For this review, take the finished solid that the model builds, in its own axes (mm). Face numbers are marked on the shaded views. A direction names the side the tool comes from. Coordinates: 2 decimals unless noted, no trailing zeros. Loops run counter-clockwise (first coordinate to the right, second up) from the corner with the lowest first, then second, coordinate; pieces in that order, holes last. Notation, with made-up numbers: M 41.25,29.5 L 62.25,29.5 A8 ccw 62.25,39.5 Z; hole C 77.25,-16 d4. An arc over 180 degrees is marked long. Use one line per item in the form item = value.
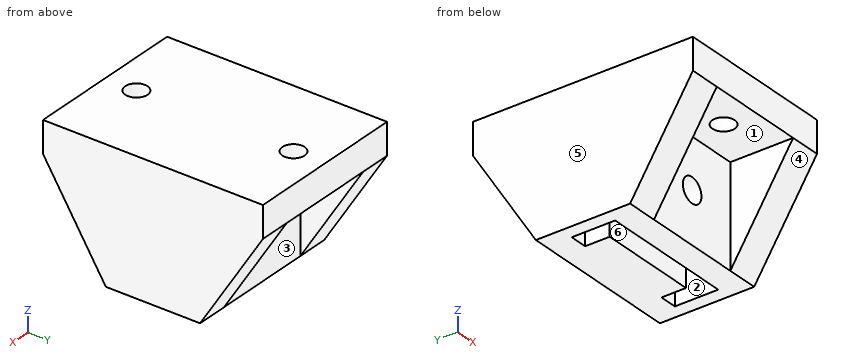
```python
from build123d import *

# Parameters (mm, degrees)
ESQUISSE1_W             = 33.02
ESQUISSE1_H             = 19.05
BOSS_EXTRU_1_DEPTH      = 20.32
ESQUISSE2_R             = 2.4765
ENL_V_MAT_EXTRU_1_DEPTH = 33.378773911
ESQUISSE3_W             = 33.02
ESQUISSE3_H             = 44.45
BOSS_EXTRU_2_DEPTH      = 6.35
BOSS_EXTRU_3_DEPTH      = 6.35
ESQUISSE6_R             = 2.25
ENL_V_MAT_EXTRU_2_DEPTH = 35.342875899


with BuildPart() as part:
    # Esquisse1 → Boss.-Extru.1 (new body)
    with BuildSketch(Plane.XY):
        Rectangle(ESQUISSE1_W, ESQUISSE1_H)
        Polygon((-13.716, 4.3815), (-13.716, -4.3815), (13.716, -4.3815), (13.716, 4.3815), (10.16, 4.3815), (10.16, -0.5715), (-10.16, -0.5715), (-10.16, 4.3815), align=None, mode=Mode.SUBTRACT)
    extrude(amount=BOSS_EXTRU_1_DEPTH)

    # Esquisse2 → Enlèv. mat.-Extru.1 (cut, through all)
    with BuildSketch(Plane(origin=(0, 9.525, 0), x_dir=(1, 0, 0), z_dir=(0, 1, 0))):
        with Locations(Location((0, -10.287, 0), (0, 0, 270))):
            Circle(ESQUISSE2_R)
    extrude(amount=-ENL_V_MAT_EXTRU_1_DEPTH, mode=Mode.SUBTRACT)

    # Esquisse3 → Boss.-Extru.2 (add)
    with BuildSketch(Plane.XY.offset(20.32)):
        Rectangle(ESQUISSE3_W, ESQUISSE3_H)
    extrude(amount=BOSS_EXTRU_2_DEPTH)

    # Esquisse5 → Boss.-Extru.3 (add)
    with BuildSketch(Plane(origin=(16.51, 0, 0), x_dir=(0, 0, -1), z_dir=(1, 0, 0))):
        Polygon((-20.32, -22.225), (0, -9.525), (-20.32, -9.525), align=None)
        Polygon((-20.32, 22.225), (0, 9.525), (-20.32, 9.525), align=None)
    boss_extru_3 = extrude(amount=-BOSS_EXTRU_3_DEPTH)

    # Symétrie1: Boss.-Extru.3 across plane
    add(boss_extru_3.mirror(Plane(origin=(0, 0, 0), x_dir=(0, 0, 1), z_dir=(1, 0, 0))))

    # Esquisse6 → Enlèv. mat.-Extru.2 (cut, through all)
    with BuildSketch(Plane(origin=(0, 0, 20.32), x_dir=(-1, 0, 0), z_dir=(0, 0, -1))):
        with Locations((0, -15.875)):
            Circle(ESQUISSE6_R)
        with Locations(Location((0, 15.875, 0), (0, 0, 180))):
            Circle(ESQUISSE6_R)
    extrude(amount=-ENL_V_MAT_EXTRU_2_DEPTH, mode=Mode.SUBTRACT)


solid = part.part
```
1. Consider section B-B on y = 2. Write out the cut boundary in (x, z).
Computed values:
outline = M -16.51,0 L -13.72,0 L -13.72,20.32 L -10.16,20.32 L -10.16,0 L 10.16,0 L 10.16,20.32 L 13.72,20.32 L 13.72,0 L 16.51,0 L 16.51,26.67 L -16.51,26.67 Z; hole C 0,10.29 d4.95
2. Consider section D-D on x = -13. Write out the cut boundary in (y, z) (1 decimal), plus the area to 3 significant figures.
Computed values:
outline = M -22.2,20.3 L -9.5,0 L -4.4,0 L -4.4,20.3 L 4.4,20.3 L 4.4,0 L 9.5,0 L 22.2,20.3 L 22.2,26.7 L -22.2,26.7 Z
area = 749 mm2
3. Consider section A-A on x = 0. Write out the cut boundary in (y, z) (1 decimal), plus the area to 3 significant figures.
Computed values:
outline = M -22.2,20.3 L -18.1,20.3 L -18.1,26.7 L -22.2,26.7 Z; M -13.6,20.3 L -9.5,20.3 L -9.5,12.8 L -4.4,12.8 L -4.4,20.3 L -0.6,20.3 L -0.6,12.8 L 9.5,12.8 L 9.5,20.3 L 13.6,20.3 L 13.6,26.7 L -13.6,26.7 Z; M -9.5,0 L -4.4,0 L -4.4,7.8 L -9.5,7.8 Z; M -0.6,0 L 9.5,0 L 9.5,7.8 L -0.6,7.8 Z; M 18.1,20.3 L 22.2,20.3 L 22.2,26.7 L 18.1,26.7 Z
area = 459 mm2
4. For pin 1 Ø4.5 at (x, z) = (0, 10.287) entering from +Y; pin 2 Ø10 at (x, z) = (1.5, 14.5) entering from -Y (3 decimals); pin 3 Ø2 at (x, y) = (6, 13) entering from -Z; pin 4 Ø1.5 at (x, z) = (9, 19) entering from +Y (3 decimals), all flat-tipped, find the tip position at first contact; note any pin that passes through.
Computed values:
pin_1 = through
pin_2 = -9.525
pin_3 = 20.32
pin_4 = 9.525
5. Wall thickness on line 1 along Y through (x, z) = (0, 23.75) (3 decimals); line 2 along X through (y, z) = (3.5, 3.75); line 3 along X through (y, z) = (13.5, 9.5): over which ranges is each line inside the solid? List them lowest first. Write a range as from..to.
Computed values:
line_1 = -22.225..-18.125, -13.625..13.625, 18.125..22.225
line_2 = -16.51..-13.72, -10.16..10.16, 13.72..16.51
line_3 = -16.51..-10.16, 10.16..16.51
6. Tool access review of the marked faces 1, 2 and 3: name each direction out of +Z, -Z, +X, -X, +Y, -Y from which nothing blocks a thin tool from reaching the whole face with its end or side.
Computed values:
face_1 = -Z, -Y
face_2 = -Z
face_3 = -Z, +Y
7. Draft analysis for pull direction Y (two halves, no side actions). For the marked faces 4, 5 and 6, state which applies: +Y half, -Y half, draft (parallel to the pull), parting line (faces both ways), or undercut.
Computed values:
face_4 = -Y half
face_5 = draft
face_6 = undercut
